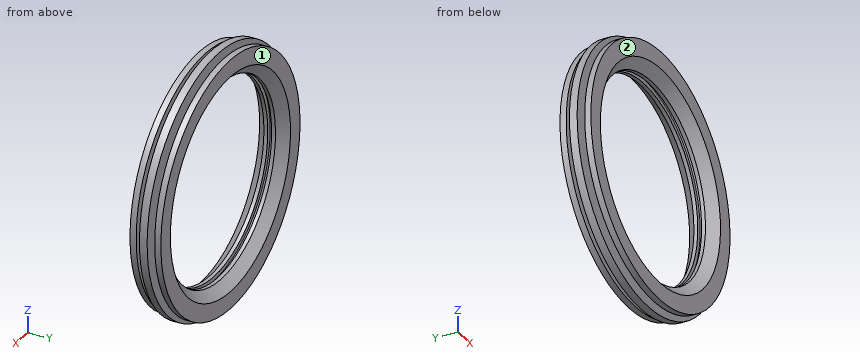
```python
from build123d import *


with BuildPart() as part:
    # Sketch1 → Revolve1 (revolve)
    with BuildSketch(Plane.XY, mode=Mode.PRIVATE) as revolve1_sk:
        with BuildLine():
            Line((40.386, 0.79375), (40.386, 2.38125))
            Line((40.386, 2.38125), (44.35475, 6.35))
            Line((44.35475, 6.35), (51.3715, 6.35))
            Line((51.3715, 6.35), (51.3715, 3.81))
            Line((51.3715, 3.81), (46.2915, 3.81))
            Line((46.2915, 3.81), (46.2915, 1.5875))
            Line((46.2915, 1.5875), (52.959, 1.5875))
            Line((52.959, 1.5875), (52.959, 0))
            Line((52.959, 0), (42.926, 0))
            ThreePointArc((42.926, 0), (42.693516008, 0.561266008), (42.13225, 0.79375))
            Line((42.13225, 0.79375), (40.386, 0.79375))
        make_face()
    revolve1 = revolve(revolve1_sk.sketch.rotate(Axis((0, 0, 0), (0, 1, 0)), 90), axis=Axis((0, 0, 0), (0, 1, 0)))

    # Mirror1: Revolve1 across plane
    add(revolve1.mirror(Plane.ZX))


solid = part.part
```
Read the model definition and answer for the solid it produces. Units are mm, in the model's axes. Face numbers are marked on the shaded views. Give positions to 0.01 mm unless a question says otherwise; leave off trailing zeros. Put each result on its own line as item: value. Start each with the question number.
1. Consider line 1 along Y through (x, z) = (-46, -13.5); line 2 along X through (y, z) = (1.4, 0); line 3 along X through (y, z) = (4.75, 37.5). Determine where each line is inside the solid, lowest interval first.
2. Each of these flat-tipped pins is pushed along its axis until it touches: pin 1 Ø10 at (x, z) = (-38.5, 7) entering from +Y; pin 2 Ø6 at (x, y) = (-42, -3.5) entering from -Z; pin 3 Ø1 at (y, z) = (4.5, 26.5) entering from +X. Where does it stop, or does it pass through?
3. For a pull along Y with two mould halves and no side action, classify the marked faces 1 and 2 as released by +Y, released by -Y, zero draft, split by the parting line, or undercut.
Final values:
1. line 1: y = -6.35 to -3.81, -1.59 to 1.59, 3.81 to 6.35
1. line 2: x = -52.96 to -40.39, 40.39 to 52.96
1. line 3: x = -35.11 to -20.54, 20.54 to 35.11
2. pin 1: stops at y = 6.13
2. pin 2: stops at z = -35.06
2. pin 3: stops at x = 44.31
3. face 1: released by +Y
3. face 2: released by -Y
